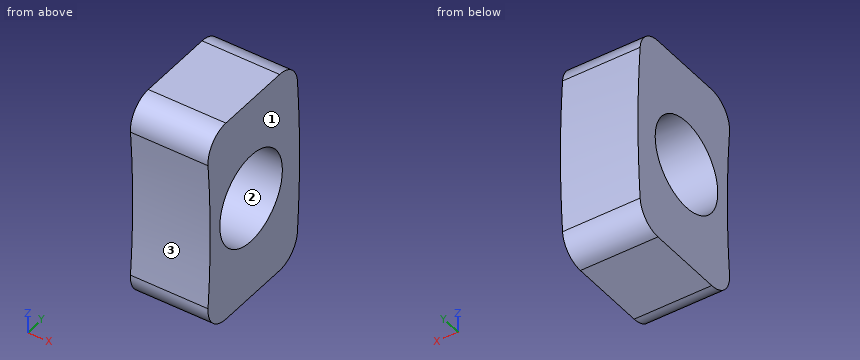
Autodesk Inventor part; units mm, degrees
ref_plane "YZ Plane" through (0, 0, 0) normal (1, 0, 0) x (0, 1, 0)
ref_plane "XZ Plane" through (0, 0, 0) normal (0, 1, 0) x (-1, 0, 0)
ref_plane "XY Plane" through (0, 0, 0) normal (0, 0, 1) x (1, 0, 0)
sketch "Sketch1" plane through (0, 0, 0) normal (1, 0, 0) x (0, 1, 0)
  circle A0 centre (0, 0) radius 43.75 construction
  circle A1 centre (0, 0) radius 38.75 construction
  line L0 (48.236, 0) -> (48.236, 4) construction
  line L1 (48.236, 0) -> (48.236, -4) construction
  arc A2 (43.5668, -4) -> (43.5668, 4) centre (0, 0) ccw construction
  arc A3 (38.543, -4) -> (38.543, 4) centre (0, 0) ccw construction
  line L2 (43.5668, 4) -> (38.543, 4)
  line L3 (38.543, -4) -> (43.5668, -4)
  arc A4 (38.543, -4) -> (38.543, 4) centre (3.2648, 0) ccw
  arc A5 (43.5668, -4) -> (43.5668, 4) centre (3.2648, 0) ccw
  line L4 (38.769, 0) -> (43.7648, 0) construction
  line L5 (41.0549, 4) -> (41.0549, -4) construction
  circle A6 centre (41.0549, 0) radius 1.75 construction
  circle A7 centre (41.0549, 0) radius 1.75
  dimension "d0" = 87.5
  dimension "d1" = 77.5
  dimension "d2" = 4
  dimension "d3" = 4
  dimension "d4" = 3.5
  dimension "d5" = 3.5
  dimension "d6" = 40.5
  dimension "d7" = 7.1811
  dimension "d8" = 4
  dimension "d9" = 4
extrude "Extrusion2" add sketch "Sketch1" along normal blind 3
fillet "Fillet2" radius 1 4 edges at (1.5, 43.5668, -4) (1.5, 43.5668, 4) (1.5, 38.543, 4) (1.5, 38.543, -4)
properties part number "Reverse Gear Link Block" material "PVC-Piping"
CAD build for the part. Positions are in the model's coordinates, mm. Face numbers are marked on the shaded views. Coordinates: 2 decimals unless noted, no trailing zeros. Order: outer loops, then holes, each group sorted by start corner. A loop starts at its lowest first (then second) coordinate and runs counter-clockwise, first axis right, second up. Notation, with made-up numbers: (15, 77) - (21, 77) arc R19 cw to (21, 112) - close; hole circle Ø10 at (31.5, 7.5). An arc over 180 degrees is marked (long way). Use a Markdown table: item, result. Add a question column.
(1) Pull direction Y, two halves, no side cores. Call the marked faces 1, 2 and 3: +Y half, -Y half, draft (parallel to the pull), parting line (faces both ways), or undercut.
(2) Saw through at D-D (y = 39.1). Give the cut face in (x, z).
(3) Drill centre lines: line 1 along Z through (x, y) = (1.85, 40.65); line 2 along Z through (x, y) = (1, 42.25); line 3 along Y through (x, z) = (2.35, -1.25). Where is each one in solid material? Low to high. Write a range as [from, to].
(4) Saw through at B-B (y = 42.1). Give the cut face in (x, z), then the cut area to 3 significant figures.
(5) Saw through at A-A (z = 0). Give the cut face in (x, y).
(6) Saw through at C-C (x = 1.85). Give the cut face in (y, z).
Solved:
| question | item | result |
|---|---|---|
| 1 | face 1 | draft |
| 1 | face 2 | undercut |
| 1 | face 3 | -Y half |
| 2 | outline | (0, -3.84) - (3, -3.84) - (3, 3.84) - (0, 3.84) - close |
| 3 | line 1 | z = [-4, -1.7], [1.7, 4] |
| 3 | line 2 | z = [-4, -1.28], [1.28, 4] |
| 3 | line 3 | y = [38.75, 39.83], [42.28, 43.75] |
| 4 | outline | (0, -4) - (3, -4) - (3, -1.4) - (0, -1.4) - close; (0, 1.4) - (3, 1.4) - (3, 4) - (0, 4) - close |
| 4 | area | 15.6 mm² |
| 5 | outline | (0, 38.77) - (3, 38.77) - (3, 39.3) - (0, 39.3) - close; (0, 42.8) - (3, 42.8) - (3, 43.76) - (0, 43.76) - close |
| 6 | outline | (38.65, -2.92) arc R1 ccw to (39.65, -4) - (42.65, -4) arc R1 ccw to (43.65, -3.08) arc R40.5 ccw to (43.65, 3.08) arc R1 ccw to (42.65, 4) - (39.65, 4) arc R1 ccw to (38.65, 2.92) arc R35.5 cw to start; hole circle Ø3.5 at (41.05, 0) |
